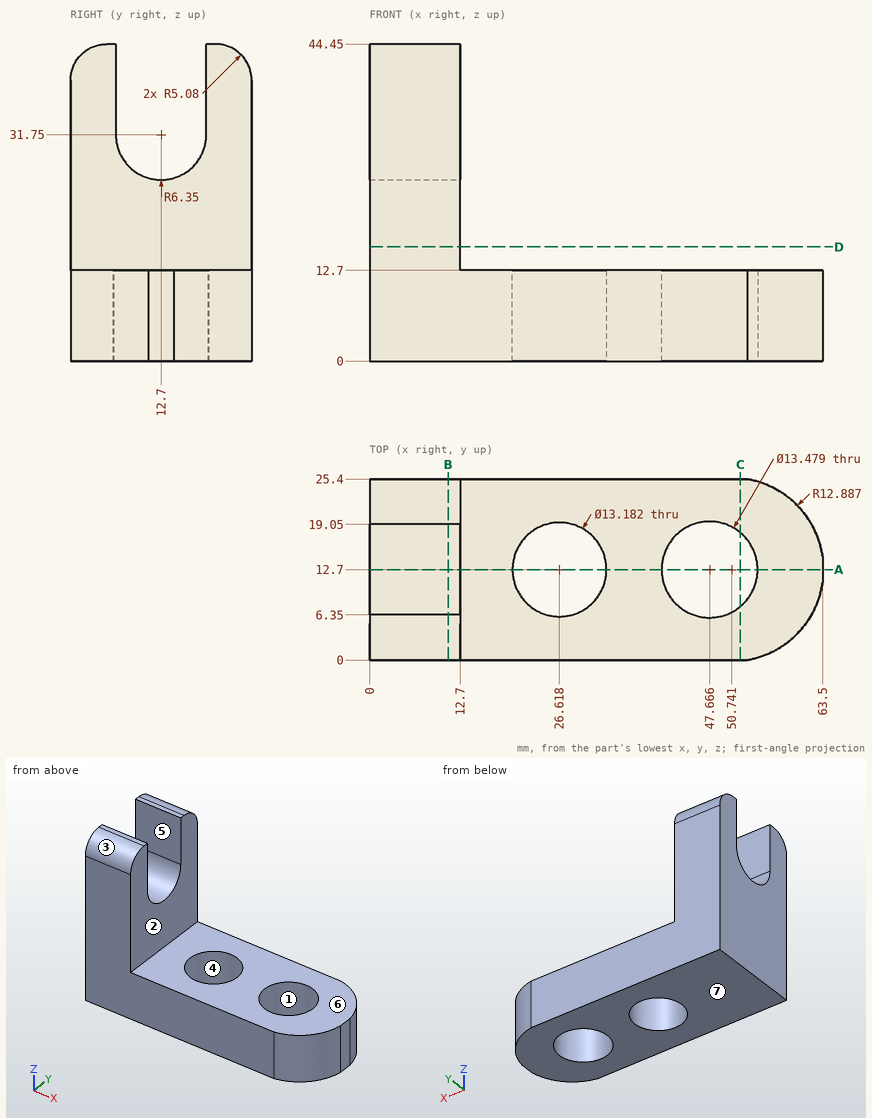
Geometry check sheet. Reference: drawing and pictorial views, mm from the part's lowest x, y, z. A direction names the side the tool comes from. Round coordinates to 2 decimals unless told otherwise and drop trailing zeros. Write each loop counter-clockwise with the first axis right and the second up, starting at its lowest first coordinate (ties: lowest second). Pieces come first, ordered by that corner, then holes. Notation, with made-up numbers: (59, -36) -> (84, -36) arc R15 cw to (84, -17) -> close; hole circle Ø9 at (27.25, 87). An arc over 180 degrees is marked (long way). Put each result on its own line as item: value.
1) Cross-section at C-C, the plane x = 52. Enter the section's corners in (y, z).
Recorded:
outline: (0, 0) -> (7.54, 0) -> (7.54, 12.7) -> (0, 12.7) -> close; (17.86, 0) -> (25.4, 0) -> (25.4, 12.7) -> (17.86, 12.7) -> close
2) Cross-section at B-B, the plane x = 11. Enter the section's corners in (y, z).
Recorded:
outline: (0, 0) -> (25.4, 0) -> (25.4, 39.37) arc R5.08 ccw to (20.32, 44.45) -> (19.05, 44.45) -> (19.05, 31.75) arc R6.35 cw to (6.35, 31.75) -> (6.35, 44.45) -> (5.08, 44.45) arc R5.08 ccw to (0, 39.37) -> close
3) Cross-section at D-D, the plane z = 16. Enter the section's corners in (x, y), plus the area to 3 significant figures.
Recorded:
outline: (0, 0) -> (12.7, 0) -> (12.7, 25.4) -> (0, 25.4) -> close
area: 323 mm2
4) Thickness scan on probe 1 along Y at (x, z) = (7.5, 33); probe 2 along Y at (x, z) = (47.5, 12.5); probe 3 along X at (y, z) = (23, 36). Record the ranges inside material, lowest first. Write a range as from..to.
Recorded:
probe 1: y = 0..6.35, 19.05..25.4
probe 2: y = 0..5.96, 19.44..25.4
probe 3: x = 0..12.7
5) Cross-section at A-A, the plane y = 12.7. Enter the section's corners in (x, z) (1 decimal).
Recorded:
outline: (0, 0) -> (20, 0) -> (20, 12.7) -> (12.7, 12.7) -> (12.7, 25.4) -> (0, 25.4) -> close; (33.2, 0) -> (40.9, 0) -> (40.9, 12.7) -> (33.2, 12.7) -> close; (54.4, 0) -> (63.5, 0) -> (63.5, 12.7) -> (54.4, 12.7) -> close
6) Access from +Z, -Z, +X, -X, +Y, -Y to the whole of each face (thin tool, end or side, straight path). Record for the marked faces 5, 6 and 7.
Recorded:
face 5: +Z, +X, -X
face 6: +Z, +X, +Y, -Y
face 7: -Z, +X, -X, +Y, -Y
7) Release check for a two-part mould opening along X. For the marked faces 1, 2, 3 and 4 record: pulls with the +X half, pulls with the -X half, needs draft (parallel to the pull), parting line crosses it, or undercut.
Recorded:
face 1: undercut
face 2: pulls with the +X half
face 3: needs draft
face 4: undercut
8) Depth check by flat-ended pin: P1, Ø5, axis at y = 17.5, z = 9, coming from the +X side; P2, Ø2, axis at x = 38, y = 19, coming from the +Z side; P3, Ø12.5, axis at y = 19, z = 25, coming from the +X side. Enter the tip coordinate at first touch or a pass-through.
Recorded:
P1: stops at x = 63.42
P2: stops at z = 12.7
P3: stops at x = 12.7
